Could you check a few things on this drawing? It's one solid part, dimensions in mm from its lowest x, y, z. Give positions to 0.01 mm unless a question says otherwise; leave off trailing zeros. Order: outer loops, then holes, each group sorted by start corner. A loop starts at its lowest first (then second) coordinate and runs counter-clockwise, first axis right, second up.
Item 1: I want a section at D-D, the plane x = 128.5. Write out the boundary of the cut face in (y, z).
Item 2: If I drill on line 1 along X through (y, z) = (4.25, 85) (1 decimal); line 2 along Z through (x, y) = (129.5, 5) (1 decimal); line 3 along Z through (x, y) = (317, 1.5) (1 decimal), over which ranges is the centre line in solid material (lowest first)?
Item 3: I want a section at B-B, the plane y = 3.25. Count the separate pieces of the cut face and the enclosed holes in it.
Item 4: I'm going to push a flat-ended pin straight in: pin 1 Ø3 at (x, y) = (288.5, 2) entering from -Z (1 decimal). Where does the tip first touch, or does it pass through?
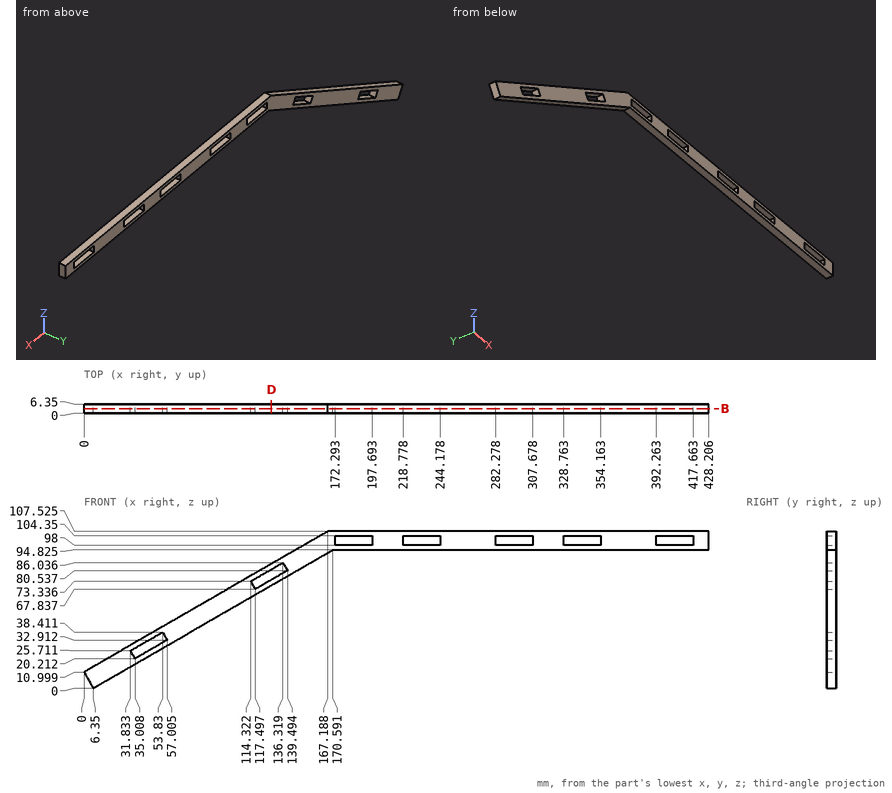
Results list:
1. outline: (0, 70.52) - (6.35, 70.52) - (6.35, 74.19) - (0, 74.19) - close; (0, 81.52) - (6.35, 81.52) - (6.35, 85.19) - (0, 85.19) - close
2. line 1: x = 128.2 to 134.5, 136.9 to 153.6
2. line 2: z = 71.1 to 74.8, 82.1 to 85.8
2. line 3: z = 94.8 to 107.5
3. separate pieces: 1
3. enclosed holes: 7
4. pin 1: stops at z = 94.8
